Verification items for the finished model (mm, model axes). A direction names the side the tool comes from. Coordinates: 2 decimals unless noted, no trailing zeros. Order: outer loops, then holes, each group sorted by start corner. A loop starts at its lowest first (then second) coordinate and runs counter-clockwise, first axis right, second up. Notation, with made-up numbers: M 75,-8.75 L 91,-8.75 A8 cw 91,-4.75 Z; hole C 79,17.5 d1. An arc over 180 degrees is marked long. Return JSON: item names as keys, results as strings.
```python
from build123d import *

# Parameters (mm, degrees)
SZKIC1_W                    = 8
SZKIC1_H                    = 1.995325655
DODANIE_WYCI_GNI_CIE1_DEPTH = 15
SZKIC3_W                    = 5
SZKIC3_H                    = 1.995325655
DODANIE_WYCI_GNI_CIE2_DEPTH = 2
SZKIC5_W                    = 5
SZKIC5_H                    = 1.995325655
DODANIE_WYCI_GNI_CIE3_DEPTH = 2


with BuildPart() as part:
    # Szkic1 → Dodanie-wyciągnięcie1 (new body)
    with BuildSketch(Plane.XY):
        with Locations((-4, -374.322437992)):
            Rectangle(SZKIC1_W, SZKIC1_H)
    extrude(amount=-DODANIE_WYCI_GNI_CIE1_DEPTH)

    # Szkic3 → Dodanie-wyciągnięcie2 (add)
    with BuildSketch(Plane.ZY.offset(8)):
        with Locations((-7.5, -374.322437992)):
            Rectangle(SZKIC3_W, SZKIC3_H)
    extrude(amount=DODANIE_WYCI_GNI_CIE2_DEPTH)

    # Szkic5 → Dodanie-wyciągnięcie3 (add)
    with BuildSketch(Plane(origin=(0, 0, 0), x_dir=(0, 0, -1), z_dir=(1, 0, 0))):
        with Locations((7.5, -374.322437992)):
            Rectangle(SZKIC5_W, SZKIC5_H)
    extrude(amount=DODANIE_WYCI_GNI_CIE3_DEPTH)


solid = part.part
```
Q1. Tool access check on faces 1 (the face through (-8, -374, -2)), 2 (the face through (1, -374, -5)), 3 (the face through (-8, -374, -12)), 4 (the face through (1, -374, -10)). Record the directions out of +Z, -Z, +X, -X, +Y, -Y that give a thin tool (end or side, any length) a straight path to the whole face; none if there is none.
Values:
{"face 1": "+Z, -X, +Y, -Y", "face 2": "+Z, +X, +Y, -Y", "face 3": "-Z, -X, +Y, -Y", "face 4": "-Z, +X, +Y, -Y"}
Q2. Cross-section at A-A, the plane y = -373.95. Record the boundary of the cut face in (x, z), and give its area (3 significant figures).
Values:
{"outline": "M -10,-10 L -8,-10 L -8,-15 L 0,-15 L 0,-10 L 2,-10 L 2,-5 L 0,-5 L 0,0 L -8,0 L -8,-5 L -10,-5 Z", "area": "140 mm^2"}
Q3. Material ranges on line 1 along X through (y, z) = (-373.8, -12.75); line 2 along Z through (x, y) = (-9, -374.25), recorded low to high.
Values:
{"line 1": "-8 to 0", "line 2": "-10 to -5"}
Q4. Cross-section at B-B, the plane x = 0.25. Record the boundary of the cut face in (y, z).
Values:
{"outline": "M -375.32,-10 L -373.32,-10 L -373.32,-5 L -375.32,-5 Z"}
Q5. Go/stop test with flat-tipped pins: pin 1 (0.6 mm diameter, centred on y = -374.5, z = -12, fed in from +X); pin 2 (0.6 mm diameter, centred on x = -9, y = -374.5, fed in from +Z); pin 3 (0.6 mm diameter, centred on x = -9, y = -374, fed in from -Z). Record where each tip stops, or that it passes through.
Values:
{"pin 1": "x = 0", "pin 2": "z = -5", "pin 3": "z = -10"}
Q6. Cross-section at C-C, the plane z = -13. Record the boundary of the cut face in (x, y).
Values:
{"outline": "M -8,-375.32 L 0,-375.32 L 0,-373.32 L -8,-373.32 Z"}
